Design review of the part built by this model. Coordinates are the model's own, in mm. A direction names the side the tool comes from. Coordinates: 2 decimals unless noted, no trailing zeros. Write each loop counter-clockwise with the first axis right and the second up, starting at its lowest first coordinate (ties: lowest second). Pieces come first, ordered by that corner, then holes. Notation, with made-up numbers: (-39, -33) - (-7, -33) arc R21 ccw to (-7, 0) - close; hole circle Ø5 at (28, -28.5). An arc over 180 degrees is marked (long way). Answer as a JSON object with one key per item and string values.
Autodesk Inventor part; units mm, degrees
ref_plane "YZ Plane" through (0, 0, 0) normal (1, 0, 0) x (0, 1, 0)
ref_plane "XZ Plane" through (0, 0, 0) normal (0, 1, 0) x (-1, 0, 0)
ref_plane "XY Plane" through (0, 0, 0) normal (0, 0, 1) x (1, 0, 0)
sketch "Sketch1" plane through (0, 0, 0) normal (0, 0, 1) x (1, 0, 0)
  circle A0 centre (0, 0) radius 1.7526
  dimension "d0" = 3.5052
extrude "Extrusion1" add sketch "Sketch1" along normal blind 25.4
sketch "Sketch2" plane through (0, 0, 25.4) normal (0, 0, 1) x (1, 0, 0)
  line L0 (-2.8702, 2.8702) -> (2.8702, 2.8702)
  line L1 (2.8702, 2.8702) -> (2.8702, -2.8702)
  line L2 (2.8702, -2.8702) -> (-2.8702, -2.8702)
  line L3 (-2.8702, -2.8702) -> (-2.8702, 2.8702)
  point P0 (0, 0)
  dimension "d3" = 5.7404
  dimension "d4" = 5.7404
  dimension "d5" = 2.8702
  dimension "d6" = 2.8702
  dimension "d7" = 2.8702
extrude "Extrusion2" add sketch "Sketch2" along normal blind 2.54
thread "Thread1"
(1) To check wall thickness, follow line 1 (Z direction, x = 0, y = 2.35); line 2 (X direction, y = 0.9, z = 3.25); line 3 (X direction, y = 1.3, z = 18.5). State the ranges of each line that lie inside material, in increasing order. Write a range as from..to.
Solved:
{"line 1": "z = 25.4..27.94", "line 2": "x = -1.5..1.5", "line 3": "x = -1.18..1.18"}
(2) Tool access review of faces 1 (the face through (0, 2, 25.4)), 2 (the face through (0, -2.87, 27)): name each direction out of +Z, -Z, +X, -X, +Y, -Y from which nothing blocks a thin tool from reaching the whole face with its end or side.
Solved:
{"face 1": "-Z", "face 2": "+Z, -Z, +X, -X, -Y"}
(3) Take a section at A-A, the plane x = 0. Write out the cut boundary in (y, z).
Solved:
{"outline": "(-2.87, 25.4) - (-1.75, 25.4) - (-1.75, 0) - (1.75, 0) - (1.75, 25.4) - (2.87, 25.4) - (2.87, 27.94) - (-2.87, 27.94) - close"}
(4) Take a section at C-C, the plane z = 23. Write out the cut boundary in (x, y), and give its area (3 significant figures).
Solved:
{"outline": "circle Ø3.51 at (0, 0)", "area": "9.65 mm^2"}
(5) For pin 1 (1 mm diameter, centred on y = -0.5, z = 5, fed in from -X); pin 2 (1.5 mm diameter, centred on y = -1, z = 22.5, fed in from -X); pin 3 (1 mm diameter, centred on y = -1.5, z = 16, fed in from -X), all flat-tipped, find the tip position at first contact; note any pin that passes through.
Solved:
{"pin 1": "stops at x = -1.75", "pin 2": "stops at x = -1.73", "pin 3": "stops at x = -1.44"}
(6) Take a section at D-D, the plane y = -2.35. Write out the cut boundary in (x, z).
Solved:
{"outline": "(-2.87, 25.4) - (2.87, 25.4) - (2.87, 27.94) - (-2.87, 27.94) - close"}
